Here's how the part is built. I have some questions about the finished solid (model axes, mm). A direction names the side the tool comes from. Round coordinates to 2 decimals unless told otherwise and drop trailing zeros. Loops run counter-clockwise (first coordinate to the right, second up) from the corner with the lowest first, then second, coordinate; pieces in that order, holes last. Notation, with made-up numbers: (31, -13.5) -> (51, -13.5) arc R27 cw to (51, 15.5) -> close; hole circle Ø3 at (-19.75, 44). An arc over 180 degrees is marked (long way). One line per item, written item: value. Start each with the question number.
```python
from build123d import *

# Parameters (mm, degrees)
F1_DEPTH = 63.5
F0_W     = 25.4
F0_H     = 19.05
F2_DEPTH = 25.4
F3_DEPTH = 7.9375
F5_R     = 6.35
F6_R     = 11.1630975277
F7_DEPTH = 35


with BuildPart() as f1:
    # F0 (on Front) → F1 (new body, symmetric)
    with BuildSketch(Plane.XZ):
        Polygon((22.225, 9.525), (-41.275, 9.525), (-41.275, -9.525), (41.275, -9.525), (41.275, 9.525), align=None)
    extrude(amount=F1_DEPTH, both=True)

    # F0 (on Front) → F2 (join, symmetric)
    with BuildSketch(Plane.XZ):
        with BuildLine():
            Line((22.225, 27.0002), (22.225, 9.525))
            Line((22.225, 9.525), (41.275, 9.525))
            Line((41.275, 9.525), (41.275, 27.0002))
            ThreePointArc((41.275, 27.0002), (45.9246798487, 38.2255201513), (57.15, 42.8752))
            Line((57.15, 42.8752), (60.325, 42.8752))
            Line((60.325, 42.8752), (60.325, 61.9252))
            Line((60.325, 61.9252), (57.15, 61.9252))
            ThreePointArc((57.15, 61.9252), (32.4542956671, 51.6959043329), (22.225, 27.0002))
        make_face()
        with Locations((73.025, 52.4002)):
            Rectangle(F0_W, F0_H)
    extrude(amount=F2_DEPTH, both=True)

    # F0 (on Front) → F3 (join, symmetric)
    with BuildSketch(Plane.XZ):
        with BuildLine():
            add(Edge.make_bspline(
                [(-41.275, 9.525), (-41.275, 45.1444163918), (8.36633984, 62.1046647429), (57.15, 61.9252)],
                knots=[0, 0, 0, 0, 111.5045361635, 111.5045361635, 111.5045361635, 111.5045361635], degree=3))
            Line((-41.275, 9.525), (22.225, 9.525))
            Line((22.225, 9.525), (22.225, 27.0002))
            ThreePointArc((22.225, 27.0002), (32.4542956671, 51.6959043329), (57.15, 61.9252))
        make_face()
    extrude(amount=F3_DEPTH, both=True)

    # F0 (on Front) → F4 (revolve)
    with BuildSketch(Plane.XZ):
        Polygon((85.725, 62.9158), (85.725, 61.9252), (85.725, 42.8752), (85.725, 31.1658), (111.125, 31.1658), (111.125, 62.9158), align=None)
    revolve(axis=Axis((85.725, 0, 47.0408), (0, 0, 1)))

    # F5
    f5_edges = [f1.edges().sort_by_distance(p)[0] for p in [
        (41.275, 63.5, 0),
        (-41.275, 63.5, 0),
        (-41.275, -63.5, 0),
        (41.275, -63.5, 0),
    ]]
    fillet(f5_edges, radius=F5_R)

    # F6 (on face) → F7 (cut)
    with BuildSketch(Plane.XY.offset(62.9158)):
        with Locations((85.725, 0)):
            Circle(F6_R)
    extrude(amount=-F7_DEPTH, mode=Mode.SUBTRACT)


solid = f1.part
```
Q1. I want a section at A-A on y = -36. Please give me the cut outline in (x, z) (3 decimals).
Q2. If I drill on line 1 along Z through (x, y) = (-15.5, 18) (3 decimals); line 2 along Y through (x, z) = (94, 46.5); line 3 along Y through (x, z) = (25.5, 32.5), over which ranges is the centre line in solid material (lowest first)?
Q3. Will these pins go through, and if not, where does the flat tip stop? P1, Ø18.5, axis at y = -14, z = 5, coming from the +X side (3 decimals); P2, Ø1, axis at x = 53.5, y = -8.5, coming from the -Z side; P3, Ø4, axis at x = 9, y = 45.5, coming from the +Z side (3 decimals).
Q4. I want a section at B-B on y = -17. Please give me the cut outline in (x, z) (3 decimals), plus the area to 3 significant figures.
Q5. Which directions (+Z, -Z, +X, -X, +Y, -Y) give clear straight access to the entire face, cutting with the end or side of a thin tool? Please do faces 5 (the flat face through (46, -25.4, 42)), 6 (the flat face through (46, 25.4, 42)), 7 (the flat face through (60, -2, 61.925)), 8 (the cylindrical face through (32.73, 16.55, 51.97)).
Q6. If we mould it in two halves opening along X, with no side actions, what happens to faces 1 (the cylindrical face through (109.2, -9.7, 43.7)), 2 (the cylindrical face through (-39.365, -61.689, -0.133)), 3 (the flat face through (1, -36, 9.525)), 4 (the cylindrical face through (45.8, -0.4, 38.1))? For each: released by +X, released by -X, zero draft, split by the parting line, or undercut.
Answers below:
1. outline: (-41.275, -9.525) -> (41.275, -9.525) -> (41.275, 9.525) -> (-41.275, 9.525) -> close
2. line 1: z = -9.525 to 9.525
2. line 2: y = -24.01 to -7.49, 7.49 to 24.01
2. line 3: y = -25.4 to 25.4
3. P1: stops at x = 41.275
3. P2: stops at z = 42.32
3. P3: stops at z = 9.525
4. outline: (-41.275, -9.525) -> (41.275, -9.525) -> (41.275, 27) arc R15.875 cw to (57.15, 42.875) -> (66.853, 42.875) -> (66.853, 31.166) -> (104.597, 31.166) -> (104.597, 62.916) -> (66.853, 62.916) -> (66.853, 61.925) -> (57.15, 61.925) arc R34.925 ccw to (22.225, 27) -> (22.225, 9.525) -> (-41.275, 9.525) -> close
4. area: 4,050 mm^2
5. face 5: +Z, +X, -X, -Y
5. face 6: +Z, +X, -X, +Y
5. face 7: +Z, -X
5. face 8: +Z, -X, +Y
6. face 1: undercut
6. face 2: released by -X
6. face 3: zero draft
6. face 4: undercut
